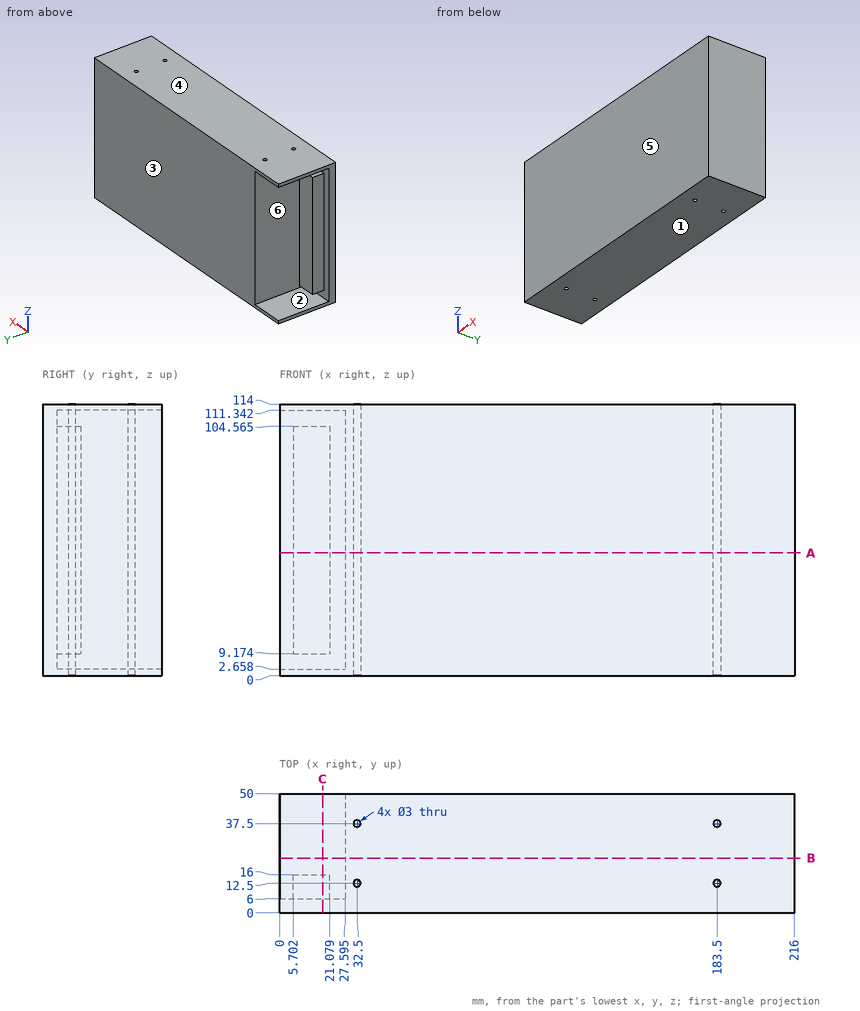
Answer from the drawing. Dimensions are ordinates in mm from the lowest x, y and z of the part. A direction names the side the tool comes from. Give positions to 0.01 mm unless a question says otherwise; leave off trailing zeros. Order: outer loops, then holes, each group sorted by start corner. A loop starts at its lowest first (then second) coordinate and runs counter-clockwise, first axis right, second up.
(1) For a pull along Z with two mould halves and no side action, classify the marked faces 1, 2, 3 and 4 as released by +Z, released by -Z, zero draft, split by the parting line, or undercut.
(2) Given pin 1 (2 mm diameter, centred on x = 31.5, y = 24, fed in from -Z); pin 2 (8.5 mm diameter, centred on x = 15.5, z = 34, fed in from +Y); pin 3 (13 mm diameter, centred on y = 31, z = 40.5, fed in from -X) (3 decimals); pin 4 (5 mm diameter, centred on y = 14, z = 66, fed in from -X), each flat-ended and moving along its own axis, determine where each tip first touches the part or whether it passes through.
(3) Straight lines are drawn through the part: L1, parallel to Y at x = 32.5, z = 65; L2, parallel to X at y = 10, z = 23.5 (1 decimal); L3, parallel to Z at x = 11, y = 36.5. For each, find the intervals that lie inside material, in ascending order.
(4) For the marked faces 5 and 6, determine the directions among +Z, -Z, +X, -X, +Y, -Y from which every point of the face is accessible in a straight line to the end or side of a thin tool.
(5) Find section B-B (y = 23). Give the vertices of the cut face in (x, z) (1 decimal).
(6) Find section A-A (z = 51.5). Give the vertices of the cut face in (x, y) (1 decimal).
(7) Find section C-C (x = 18). Give the vertices of the cut face in (y, z) (1 decimal).
Result sheet:
1. face 1: released by -Z
1. face 2: undercut
1. face 3: zero draft
1. face 4: released by +Z
2. pin 1: stops at z = 0
2. pin 2: stops at y = 16
2. pin 3: stops at x = 27.595
2. pin 4: stops at x = 5.7
3. L1: y = 0 to 11, 14 to 36, 39 to 50
3. L2: x = 5.7 to 21.1, 27.6 to 216
3. L3: z = 0 to 2.66, 111.34 to 114
4. face 5: +Z, -Z, +X, -X, -Y
4. face 6: +Y
5. outline: (0, 0) - (216, 0) - (216, 114) - (0, 114) - (0, 111.3) - (27.6, 111.3) - (27.6, 2.7) - (0, 2.7) - close
6. outline: (0, 0) - (216, 0) - (216, 50) - (27.6, 50) - (27.6, 6) - (21.1, 6) - (21.1, 16) - (5.7, 16) - (5.7, 6) - (0, 6) - close; hole circle Ø3 at (32.5, 12.5); hole circle Ø3 at (32.5, 37.5); hole circle Ø3 at (183.5, 12.5); hole circle Ø3 at (183.5, 37.5)
7. outline: (0, 0) - (50, 0) - (50, 2.7) - (6, 2.7) - (6, 9.2) - (16, 9.2) - (16, 104.6) - (6, 104.6) - (6, 111.3) - (50, 111.3) - (50, 114) - (0, 114) - close
